```python
from build123d import *

# Parameters (mm, degrees)
F0_R     = 30.226
F0_R_2   = 26.2509
F1_DEPTH = 1695.45
F3_DEPTH = 103.124
F5_DEPTH = 124.968


with BuildPart() as f1:
    # F0 (on Top) → F1 (new body)
    with BuildSketch(Plane.XY):
        with Locations((-125.815094, -56.057207)):
            Circle(F0_R)
        with Locations((-125.815094, -56.057207)):
            Circle(F0_R_2, mode=Mode.SUBTRACT)
    extrude(amount=F1_DEPTH)

    # F2 (on Front) → F3 (cut)
    with BuildSketch(Plane.XZ):
        Polygon((-89.987062, 69.129817), (-159.116879, 0), (-88.816114, 0), align=None)
    extrude(amount=F3_DEPTH, mode=Mode.SUBTRACT)

    # F4 (on Front) → F5 (cut)
    with BuildSketch(Plane.XZ):
        Polygon((-93.407938, 1702.409625), (-163.886861, 1702.409625), (-93.407938, 1631.930702), align=None)
    extrude(amount=F5_DEPTH, mode=Mode.SUBTRACT)


solid = f1.part
```
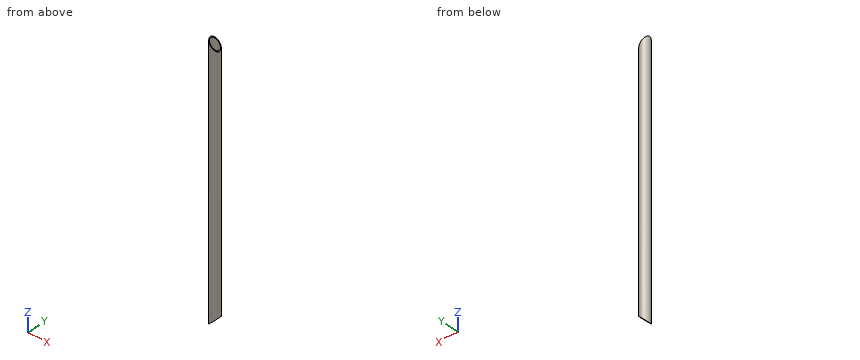
Geometry: final body of the model. Coordinates: model frame, mm. Round coordinates to 2 decimals unless told otherwise and drop trailing zeros. Loops run counter-clockwise (first coordinate to the right, second up) from the corner with the lowest first, then second, coordinate; pieces in that order, holes last.
Item 1: Contact query for flat-ended pins moving along their axis: P1, Ø6, axis at y = -47, z = 1097.5, coming from the -X side; P2, Ø3, axis at x = -147, z = 1383.5, coming from the -Y side; P3, Ø1, axis at x = -145.5, z = 845, coming from the +Y side. Output: stop coordinate, or through.
Checked values:
P1: stops at x = -155.43
P2: stops at y = -78.99
P3: stops at y = -32.7
Item 2: Section B-B, the plane y = -71.5. Output: boundary loops of the cut face in (x, z).
Checked values:
outline: (-151.8, 7.32) - (-147.04, 12.07) - (-147.04, 1685.57) - (-151.8, 1690.32) - close; (-104.59, 54.53) - (-99.83, 59.29) - (-99.83, 1638.35) - (-104.59, 1643.11) - close
Item 3: Section A-A, the plane x = -126.5. Output: boundary loops of the cut face in (y, z).
Checked values:
outline: (-86.28, 32.62) - (-82.3, 32.62) - (-82.3, 1665.02) - (-86.28, 1665.02) - close; (-29.82, 32.62) - (-25.84, 32.62) - (-25.84, 1665.02) - (-29.82, 1665.02) - close
Item 4: Line query: L1, parallel to Y at x = -124, z = 538; L2, parallel to X at y = -60, z = 632; L3, parallel to Y at x = -129, z = 968. Output: solid intervals per line, ascending.
Checked values:
L1: y = -86.23 to -82.25, -29.87 to -25.89
L2: x = -155.78 to -151.77, -99.86 to -95.85
L3: y = -86.11 to -82.11, -30 to -26
Item 5: Section C-C, the plane z = 1578. Output: boundary loops of the cut face in (x, y).
Checked values:
outline: circle Ø60.45 at (-125.82, -56.06); hole circle Ø52.5 at (-125.82, -56.06)
